Could you check a few things on this drawing? It's one solid part, dimensions in mm from its lowest x, y, z. A direction names the side the tool comes from. Give positions to 0.01 mm unless a question says otherwise; leave off trailing zeros. Order: outer loops, then holes, each group sorted by start corner. A loop starts at its lowest first (then second) coordinate and runs counter-clockwise, first axis right, second up.
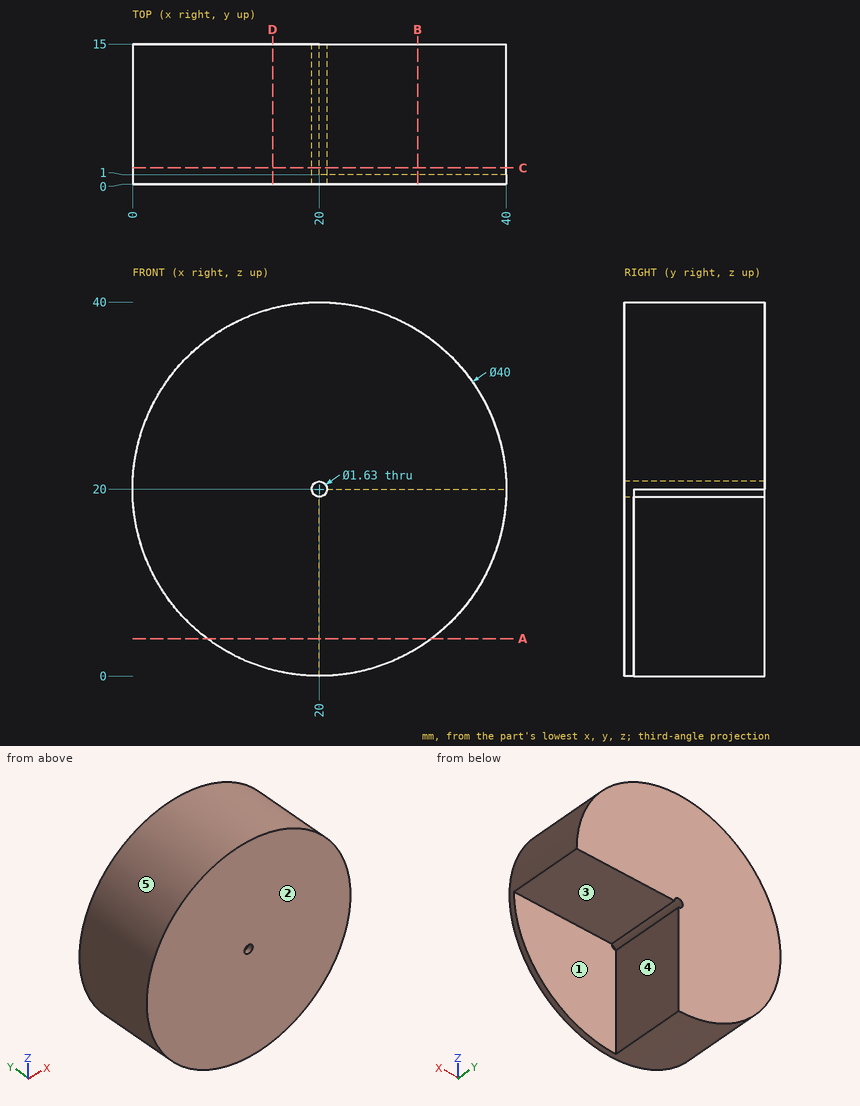
Q1. I'm going to push flat-ended pins straight in: P1, Ø7, axis at y = 6.5, z = 9, coming from the +X side; P2, Ø6, axis at x = 4.5, y = 11.5, coming from the -Z side; P3, Ø1.5, axis at x = 33, y = 7, coming from the +Z side. Where does each tip first touch, or does it pass through?
Filled sheet:
P1: stops at x = 20
P2: stops at z = 4.39
P3: stops at z = 35.81
Q2. If we section it at B-B on x = 30.5: List the corners of the cut face in (y, z) for me, plus the area to 3 significant figures.
Filled sheet:
outline: (0, 2.98) - (1, 2.98) - (1, 20) - (15, 20) - (15, 37.02) - (0, 37.02) - close
area: 272 mm2
Q3. For the marked faces 1 and 2, which set-ups out of +Z, -Z, +X, -X, +Y, -Y let a thin tool reach every point of the face, with its end or its side?
Filled sheet:
face 1: -Z, +X, +Y
face 2: +Z, -Z, +X, -X, -Y
Q4. If we section it at A-A on z = 4: List the corners of the cut face in (x, y) for me.
Filled sheet:
outline: (8, 0) - (32, 0) - (32, 1) - (20, 1) - (20, 15) - (8, 15) - close
Q5. If we section it at D-D on x = 15: List the corners of the cut face in (y, z) for me.
Filled sheet:
outline: (0, 0.64) - (15, 0.64) - (15, 39.36) - (0, 39.36) - close
Q6. Thinking about a two-plate mould opening in X: for the marked faces 3, 4 and 5, which applies, released by +X, released by -X, zero draft, split by the parting line, or undercut?
Filled sheet:
face 3: zero draft
face 4: released by +X
face 5: split by the parting line
Q7. If we section it at C-C on y = 1.75: List the corners of the cut face in (x, z) for me (3 decimals).
Filled sheet:
outline: (20, 0) - (20, 19.185) arc R0.815 cw (long way) to (20.815, 20) - (40, 20) arc R20 ccw (long way) to start
Q8. I need wall thicknesses on L1, parallel to Y at x = 38.5, z = 13; L2, parallel to X at y = 10.75, z = 19; L3, parallel to X at y = 12.25, z = 17. Which ranges of each line are inside material? Lowest first, please.
Filled sheet:
L1: y = 0 to 1
L2: x = 0.03 to 20
L3: x = 0.23 to 20
